from build123d import *

# Parameters (mm, degrees)
SKETCH1_R           = 10
BOSS_EXTRUDE1_DEPTH = 2
SKETCH2_R           = 8.5
BOSS_EXTRUDE2_DEPTH = 6
BOSS_EXTRUDE3_START = 4
SKETCH3_R           = 10
BOSS_EXTRUDE3_DEPTH = 2
SKETCH5_R           = 7
CUT_EXTRUDE2_DEPTH  = 16.362291496
BOSS_EXTRUDE4_START = 6
SKETCH6_R           = 8.875
SKETCH6_R_2         = 7
BOSS_EXTRUDE4_DEPTH = 5


with BuildPart() as part:
    # Sketch1 → Boss-Extrude1 (new body)
    with BuildSketch(Plane.XY):
        Circle(SKETCH1_R)
    extrude(amount=BOSS_EXTRUDE1_DEPTH)

    # Sketch2 → Boss-Extrude2 (add)
    with BuildSketch(Plane.XY):
        Circle(SKETCH2_R)
    extrude(amount=BOSS_EXTRUDE2_DEPTH)

    # Sketch3 → Boss-Extrude3 (add)
    with BuildSketch(Plane.XY.offset(BOSS_EXTRUDE3_START)):
        Circle(SKETCH3_R)
    extrude(amount=BOSS_EXTRUDE3_DEPTH)

    # Sketch5 → Cut-Extrude2 (cut, through all)
    with BuildSketch(Plane.XY):
        Circle(SKETCH5_R)
    extrude(amount=CUT_EXTRUDE2_DEPTH, mode=Mode.SUBTRACT)

    # Sketch6 → Boss-Extrude4 (add)
    with BuildSketch(Plane.XY.offset(BOSS_EXTRUDE4_START)):
        Circle(SKETCH6_R)
        Circle(SKETCH6_R_2, mode=Mode.SUBTRACT)
    extrude(amount=BOSS_EXTRUDE4_DEPTH)


solid = part.part
For this review, take the finished solid that the model builds, in its own axes (mm). A direction names the side the tool comes from. Round coordinates to 2 decimals unless told otherwise and drop trailing zeros. Loops run counter-clockwise (first coordinate to the right, second up) from the corner with the lowest first, then second, coordinate; pieces in that order, holes last. Notation, with made-up numbers: (41, -38.75) - (50, -38.75) arc R22 cw to (50, -29.75) - close; hole circle Ø10 at (58.25, 80). An arc over 180 degrees is marked (long way). Put each result on its own line as item: value. Start each with the question number.
1. For probe 1 along Y at (x, z) = (0, 5.5); probe 2 along Y at (x, z) = (0, 7.5) (3 decimals); probe 3 along Z at (x, y) = (6.5, 7.25), list the stretches that pass through material, from the lowest coordinate up. Write a range as [from, to].
2. Consider section C-C on z = 3.25. State the section outline as (x, y) points.
3. Insertion check: P1, Ø8, axis at x = -6.5, y = 7, coming from the +Z side; P2, Ø2, axis at y = -5, z = 6.5, coming from the -X side. Each pin has a flat end and moves straight along its axis. Give the tip position at first contact, or say it passes through.
4. Consider section A-A on x = 0. State the section outline as (y, z) points (3 decimals).
5. Consider section D-D on x = -8.25. State the section outline as (y, z) points, plus the area to 3 significant figures.
6. Mouldability with a two-part tool opening along Y and no side actions: class faces 1 (the cylindrical face through (-2.17, -9.76, 0.99)), 2 (the cylindrical face through (6.466, -2.681, 5.423)), 3 (the flat face through (7, 3, 11)) as +Y half, -Y half, draft (parallel to the pull), parting line (faces both ways), or undercut.
7. For faces 4 (the cylindrical face through (-1.924, -8.664, 8.465)), 5 (the flat face through (-4.5, -7.4, 2)), 6 (the flat face through (-7, -2, 0)), list the 3-axis set-ups (+Z, -Z, +X, -X, +Y, -Y) from which the entire face can be reached by the end or side of a thin tool; tool diameter is ignored.
Result sheet:
1. probe 1: [-10, -7], [7, 10]
1. probe 2: [-8.875, -7], [7, 8.875]
1. probe 3: [0, 2], [4, 6]
2. outline: circle Ø17 at (0, 0); hole circle Ø14 at (0, 0)
3. P1: z = 11
3. P2: x = -9.11
4. outline: (-10, 0) - (-7, 0) - (-7, 11) - (-8.875, 11) - (-8.875, 6) - (-10, 6) - (-10, 4) - (-8.5, 4) - (-8.5, 2) - (-10, 2) - close; (7, 0) - (10, 0) - (10, 2) - (8.5, 2) - (8.5, 4) - (10, 4) - (10, 6) - (8.875, 6) - (8.875, 11) - (7, 11) - close
5. outline: (-5.65, 0) - (5.65, 0) - (5.65, 2) - (2.05, 2) - (2.05, 4) - (5.65, 4) - (5.65, 6) - (3.27, 6) - (3.27, 11) - (-3.27, 11) - (-3.27, 6) - (-5.65, 6) - (-5.65, 4) - (-2.05, 4) - (-2.05, 2) - (-5.65, 2) - close
5. area: 86.1 mm^2
6. face 1: parting line
6. face 2: undercut
6. face 3: draft
7. face 4: +Z
7. face 5: none
7. face 6: -Z, +X, -X, +Y, -Y
